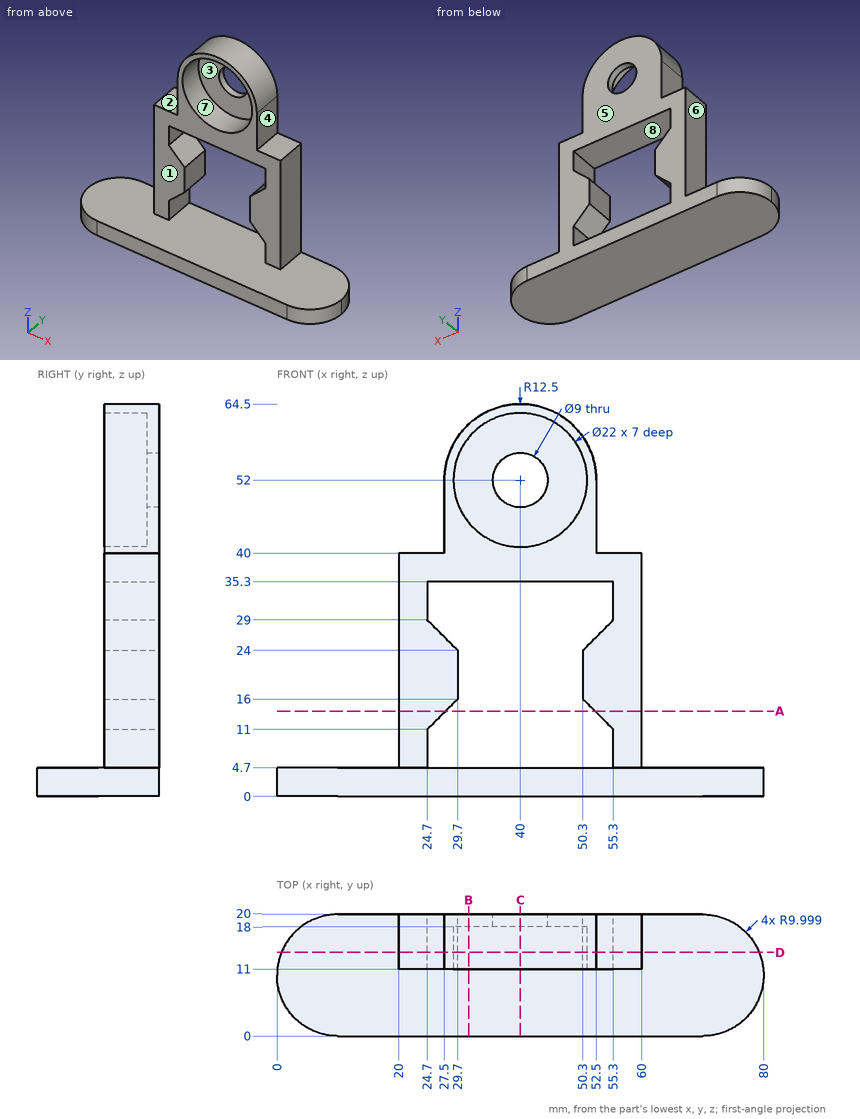
Study the drawing (mm; zero at the part's minimum x, y, z) and answer. A direction names the side the tool comes from. Give positions to 0.01 mm unless a question says otherwise; leave off trailing zeros. Loops run counter-clockwise (first coordinate to the right, second up) from the corner with the lowest first, then second, coordinate; pieces in that order, holes last. Notation, with made-up numbers: M -23.5,-29.75 L -10.5,-29.75 A29 cw -10.5,-9.75 Z; hole C -37,-10.5 d6. An arc over 180 degrees is marked long. One line per item, written item: value.
1. Section B-B on x = 31.5 is taken. Determine the outline of the cut face in (y, z), plus the area to 3 significant figures.
Found:
outline: M 0,0 L 20,0 L 20,4.7 L 0,4.7 Z; M 11,35.3 L 20,35.3 L 20,61.17 L 11,61.17 L 11,58.98 L 18,58.98 L 18,45.02 L 11,45.02 Z
area: 229 mm^2
2. Each of these flat-tipped pins is pushed along its axis until it touches: P1, Ø3, axis at y = 17, z = 7.5, coming from the +X side; P2, Ø12, axis at x = 52.5, y = 2.5, coming from the +Z side; P3, Ø2, axis at x = 44.5, y = 13.5, coming from the +Z side; P4, Ø5, axis at x = 70, y = 9, coming from the -Z side. Where does it stop, or does it pass through?
Found:
P1: x = 60
P2: z = 4.7
P3: z = 64
P4: z = 0
3. For a pull along Z with two mould halves and no side action, classify the marked faces 1, 2 and 3 as pulls with the +Z half, pulls with the -Z half, needs draft (parallel to the pull), parting line crosses it, or undercut.
Found:
face 1: needs draft
face 2: pulls with the +Z half
face 3: undercut
4. Section D-D on y = 13.75 is taken. Determine the outline of the cut face in (x, z).
Found:
outline: M 0.73,0 L 79.27,0 L 79.27,4.7 L 60,4.7 L 60,40 L 52.5,40 L 52.5,52 A12.5 ccw 27.5,52 L 27.5,40 L 20,40 L 20,4.7 L 0.73,4.7 Z; hole M 24.7,4.7 L 55.3,4.7 L 55.3,11 L 50.3,16 L 50.3,24 L 55.3,29 L 55.3,35.3 L 24.7,35.3 L 24.7,29 L 29.7,24 L 29.7,16 L 24.7,11 Z; hole C 40,52 d22
5. Section A-A on z = 14 is taken. Determine the outline of the cut face in (x, y).
Found:
outline: M 20,11 L 27.7,11 L 27.7,20 L 20,20 Z; M 52.3,11 L 60,11 L 60,20 L 52.3,20 Z
6. Section C-C on x = 40 is taken. Determine the outline of the cut face in (y, z), plus the area to 3 significant figures.
Found:
outline: M 0,0 L 20,0 L 20,4.7 L 0,4.7 Z; M 11,35.3 L 20,35.3 L 20,47.5 L 18,47.5 L 18,41 L 11,41 Z; M 11,63 L 18,63 L 18,56.5 L 20,56.5 L 20,64.5 L 11,64.5 Z
area: 185 mm^2
7. Find the intervals of material crossed by probe 1 along Z at (x, y) = (40, 18.85); probe 2 along X at (y, z) = (13.75, 23.5); probe 3 along X at (y, z) = (15.75, 8), in increasing order.
Found:
probe 1: 0 to 4.7, 35.3 to 47.5, 56.5 to 64.5
probe 2: 20 to 29.7, 50.3 to 60
probe 3: 20 to 24.7, 55.3 to 60
8. For the marked faces 4, 5, 6, 7 and 8, determine the directions among +Z, -Z, +X, -X, +Y, -Y from which every point of the face is accessible in a straight line to the end or side of a thin tool.
Found:
face 4: +Z, +X, +Y, -Y
face 5: +Z, -Z, +X, -X, +Y
face 6: +Z, -X, +Y, -Y
face 7: -Y
face 8: +Y, -Y
